Design review of the part built by this model. Coordinates are the model's own, in mm. Face numbers are marked on the shaded views. A direction names the side the tool comes from. Coordinates: 2 decimals unless noted, no trailing zeros. Loops run counter-clockwise (first coordinate to the right, second up) from the corner with the lowest first, then second, coordinate; pieces in that order, holes last. Notation, with made-up numbers: M 74,44 L 116,44 A18 ccw 116,66 Z; hole C 4,69.5 d8. An arc over 180 degrees is marked long. Answer as a JSON object with one key per item and string values. Group by question number.
1. Draft analysis for pull direction X (two halves, no side actions). For the marked faces 3, 4 and 5, state which applies: +X half, -X half, draft (parallel to the pull), parting line (faces both ways), or undercut.
2. Machinability: for the marked faces 1 and 2, which of the approach directions +Z, -Z, +X, -X, +Y, -Y give a long, thin tool a straight path to every point of the face, cutting with its end or side? Answer none if there is none.
3. Consider section D-D (x = 21). State the section outline as (y, z) points.
4. To check wall thickness, follow probe 1 along X at (y, z) = (-14, -14.5); probe 2 along Z at (x, y) = (14, -22). State the ranges of each line that lie inside material, in increasing order.
5. Consider section C-C (z = -14.5). State the section outline as (x, y) points.
6. Consider section A-A (x = 8). State the section outline as (y, z) points, then the cut area to 3 significant figures.
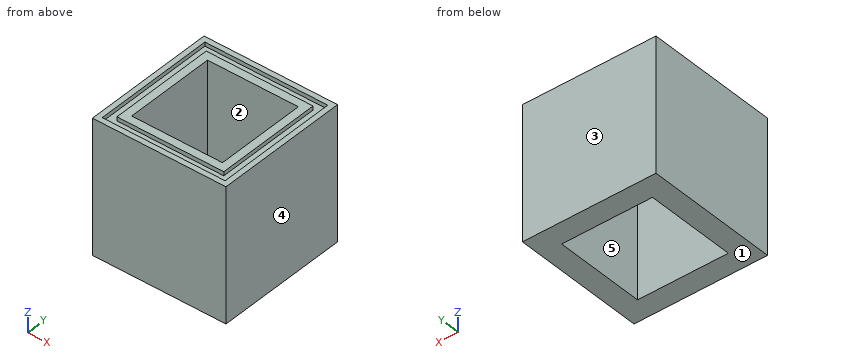
Autodesk Inventor part; units mm, degrees
ref_plane "YZ Plane" through (0, 0, 0) normal (1, 0, 0) x (0, 1, 0)
ref_plane "XZ Plane" through (0, 0, 0) normal (0, 1, 0) x (-1, 0, 0)
ref_plane "XY Plane" through (0, 0, 0) normal (0, 0, 1) x (1, 0, 0)
sketch "Esboço1" plane through (0, 0, 0) normal (0, 0, 1) x (1, 0, 0)
  line L0 (-25, -25) -> (25, -25)
  line L1 (25, -25) -> (25, 25)
  line L2 (25, 25) -> (-25, 25)
  line L3 (-25, 25) -> (-25, -25)
  line L4 (-25, -25) -> (25, 25) construction
  line L5 (25, -25) -> (-25, 25) construction
  line L6 (-17, -17) -> (17, -17)
  line L7 (17, -17) -> (17, 17)
  line L8 (17, 17) -> (-17, 17)
  line L9 (-17, 17) -> (-17, -17)
  line L10 (-17, -17) -> (17, 17) construction
  line L11 (17, -17) -> (-17, 17) construction
  point P0 (0, 0)
  dimension "d0" = 50
  dimension "d2" = 8
extrude "Extrusão1" add sketch "Esboço1" along normal mid plane 50
sketch "Esboço2" plane through (0, 0, 25) normal (0, 0, 1) x (1, 0, 0)
  line L0 (-21.5, -21.5) -> (21.5, -21.5)
  line L1 (21.5, -21.5) -> (21.5, 21.5)
  line L2 (21.5, 21.5) -> (-21.5, 21.5)
  line L3 (-21.5, 21.5) -> (-21.5, -21.5)
  line L4 (-21.5, -21.5) -> (21.5, 21.5) construction
  line L5 (21.5, -21.5) -> (-21.5, 21.5) construction
  line L6 (25, 25) -> (-25, 25)
  point P0 (0, 0)
  point P1 (0, 21.5)
  point P2 (0, -21.5)
  point P3 (-21.5, 0)
  point P4 (21.5, 0)
  dimension "d5" = 3.5
sketch "Esboço3" plane through (0, 0, 25) normal (0, 0, 1) x (1, 0, 0)
  point P0 (0, 0)
sketch "Esboço8" plane through (0, 0, 0) normal (0, 1, 0) x (-1, 0, 0)
  point P0 (0, 0)
sketch "Esboço9" plane through (0, 0, 0) normal (0, 1, 0) x (-1, 0, 0)
  line L0 (-23, 23.5) -> (-20, 23.5)
  line L1 (-20, 23.5) -> (-20, 26.5)
  line L2 (-20, 26.5) -> (-23, 26.5)
  line L3 (-23, 26.5) -> (-23, 23.5)
  line L4 (25, 25) -> (-25, 25)
  line L5 (-23, 23.5) -> (-20, 26.5) construction
  line L6 (-20, 23.5) -> (-23, 26.5) construction
  point P0 (0, 0)
  point P1 (-21.5, 25)
  dimension "d6" = 3
  dimension "d7" = 21.5
sweep "Varredura1" cut profiles "Esboço9" path "Esboço2" path curves L1 L0 L3 L2
equation "\"d3\" = d0"
properties part number "Sweep_0002_001" material "Nitreto de silício"
Findings below:
{
 "1": {"face 3": "draft", "face 4": "+X half", "face 5": "undercut"},
 "2": {"face 1": "-Z, +X, -X, +Y, -Y", "face 2": "+Z, -Z"},
 "3": {"outline": "M -25,-25 L 25,-25 L 25,25 L 23,25 L 23,23.5 L -23,23.5 L -23,25 L -25,25 Z"},
 "4": {"probe 1": "x = -25 to -17, 17 to 25", "probe 2": "z = -25 to 23.5"},
 "5": {"outline": "M -25,-25 L 25,-25 L 25,25 L -25,25 Z; hole M -17,-17 L 17,-17 L 17,17 L -17,17 Z"},
 "6": {"outline": "M -25,-25 L -17,-25 L -17,25 L -20,25 L -20,23.5 L -23,23.5 L -23,25 L -25,25 Z; M 17,-25 L 25,-25 L 25,25 L 23,25 L 23,23.5 L 20,23.5 L 20,25 L 17,25 Z", "area": "791 mm^2"}
}
